Can you work these out from the model? Positions are in its coordinate system, mm. A direction names the side the tool comes from. Coordinates: 2 decimals unless noted, no trailing zeros. Order: outer loops, then holes, each group sorted by start corner. A loop starts at its lowest first (then second) coordinate and runs counter-clockwise, first axis right, second up. Notation, with made-up numbers: (6.5, -21.75) -> (52.5, -21.75) arc R10 ccw to (52.5, -7.75) -> close; hole circle Ø9 at (38, -29). An arc over 180 degrees is marked (long way). Answer in a Markdown table with one row per item. Add a question column.
1. If I drill on line 1 along X through (y, z) = (16.75, 0); line 2 along Y through (x, z) = (54, 14.5); line 3 along X through (y, z) = (32.5, 12), over which ranges is the centre line in solid material (lowest first)? Write a range as [from, to].
2. Imagine slicing it at A-A on z = 0. Write out the boundary of the cut face in (x, y), plus the area to 3 significant figures.
3. Imagine slicing it at B-B on y = 26. Write out the boundary of the cut face in (x, z).
4. Will these pins go through, and if not, where does the flat tip stop? pin 1 (11 mm diameter, centred on y = 29.5, z = -2.5, fed in from +X); pin 2 (5.5 mm diameter, centred on x = -51.96, z = 30, fed in from +Y); pin 3 (17.5 mm diameter, centred on x = 40.5, z = 33.5, fed in from +Y); pin 4 (23 mm diameter, centred on x = 0, z = 0, fed in from -Y).
5. We'd pull the mould along Z, two halves only. Please class faces 4 (the face through (-8.99, 27.93, -22.79)), 5 (the face through (25.14, 27.93, -19.684)), 6 (the face through (17, 0, -14)): pulls with the +Z half, pulls with the -Z half, needs draft (parallel to the pull), parting line crosses it, or undercut.
6. On a 3-axis mill with a long thin cutter (end or side, diameter ignored), from which of +Z, -Z, +X, -X, +Y, -Y can I reach the whole of each face in a straight line? I mean faces 1 (the face through (-1, 11, -59)), 2 (the face through (48, 33, 33)), 3 (the face through (73, 20, 8)). Say none if no direction works.
7. Imagine slicing it at D-D on z = -40. Write out the boundary of the cut face in (x, y), plus the area to 3 significant figures.
8. Imagine slicing it at C-C on x = 28. Write out the boundary of the cut face in (y, z) (3 decimals), plus the area to 3 significant figures.
from build123d import *
from build123d.topology import SkipClean

# Parameters (mm, degrees)
SKETCH_1_W                   = 160
SKETCH_1_H                   = 118
EXTRUDE_1_DEPTH              = 23
EXTRUDE_2_DEPTH              = 38
HOLE_WIZARD_M8_2_D           = 6.8
HOLE_WIZARD_M8_2_DEPTH       = 17.957073895
HOLE_WIZARD_M8_2_CSINK_D     = 8.05
HOLE_WIZARD_M8_2_CSINK_ANGLE = 90
HOLE_WIZARD_M8_2_TIP         = 2.042926105
SKETCH_6_R                   = 24.5
EXTRUDE_3_DEPTH              = 10
EXTRUDE_4_DEPTH              = 10
SKETCH_9_R                   = 19
CUT_EXTRUDE_1_DEPTH          = 105.737767782
CUT_EXTRUDE_2_DEPTH          = 6


with BuildPart() as part:
    # Sketch 1 → Extrude 1 (new body)
    with BuildSketch(Plane(origin=(0, 0, 0), x_dir=(1, 0, 0), z_dir=(0, 1, 0))):
        Rectangle(SKETCH_1_W, SKETCH_1_H)
    extrude(amount=EXTRUDE_1_DEPTH)

    # Sketch 1_3 → Extrude 2 (add)
    with BuildSketch(Plane(origin=(0, 0, 0), x_dir=(1, 0, 0), z_dir=(0, 1, 0))):
        with BuildLine():
            ThreePointArc((-64.951905284, 37.5), (-75, 0), (-64.951905284, -37.5))
            ThreePointArc((-64.951905284, -37.5), (-44.461524227, -42.990381057), (-38.97114317, -22.5))
            ThreePointArc((-38.97114317, -22.5), (-45, 0), (-38.97114317, 22.5))
            ThreePointArc((-38.97114317, 22.5), (-44.461524227, 42.990381057), (-64.951905284, 37.5))
        make_face()
    extrude(amount=EXTRUDE_2_DEPTH)

    # Hole Wizard M8 _2
    with Locations(Plane(origin=(0, 38, 0), x_dir=(1, 0, 0), z_dir=(0, 1, 0))):
        with Locations((-51.961524227, 30), (-51.961524227, -30)):
            CounterSinkHole(HOLE_WIZARD_M8_2_D / 2, HOLE_WIZARD_M8_2_CSINK_D / 2, depth=HOLE_WIZARD_M8_2_DEPTH, counter_sink_angle=HOLE_WIZARD_M8_2_CSINK_ANGLE)
            with Locations((0, 0, -(HOLE_WIZARD_M8_2_DEPTH + HOLE_WIZARD_M8_2_TIP / 2))):  # 118° drill point
                Cone(0, HOLE_WIZARD_M8_2_D / 2, HOLE_WIZARD_M8_2_TIP, mode=Mode.SUBTRACT)

    # Sketch 6 → Extrude 3 (add)
    with BuildSketch(Plane(origin=(0, 23, 0), x_dir=(1, 0, 0), z_dir=(0, 1, 0))):
        with BuildLine():
            ThreePointArc((-16.916580755, -17.722282459), (-24.5, 0), (-16.916580755, 17.722282459))
            ThreePointArc((-16.916580755, 17.722282459), (-30.649129847, 15.709991673), (-37.095262413, 28.001435595))
            ThreePointArc((-37.095262413, 28.001435595), (-37.764179884, 25.158986305), (-38.97114317, 22.5))
            ThreePointArc((-38.97114317, 22.5), (-45, 0), (-38.97114317, -22.5))
            ThreePointArc((-38.97114317, -22.5), (-37.764179884, -25.158986305), (-37.095262413, -28.001435595))
            ThreePointArc((-37.095262413, -28.001435595), (-30.649129847, -15.709991673), (-16.916580755, -17.722282459))
        make_face()
        Circle(SKETCH_6_R)
        with BuildLine():
            Line((15, 24.5), (0, 24.5))
            ThreePointArc((0, 24.5), (17.324116139, 17.324116139), (24.5, 0))
            ThreePointArc((24.5, 0), (21.217622393, -12.25), (12.25, -21.217622393))
            Line((12.25, -21.217622393), (30, -10.969655115))
            ThreePointArc((30, -10.969655115), (32.66631784, -9.127014863), (35, -6.877903594))
            Line((35, -6.877903594), (35, 0))
            Line((35, 0), (35, 15))
            Line((35, 15), (15, 24.5))
        make_face()
    extrude(amount=EXTRUDE_3_DEPTH)

    # Sketch 8 → Extrude 4 (add)
    with BuildSketch(Plane(origin=(0, 23, 0), x_dir=(1, 0, 0), z_dir=(0, 1, 0))):
        with BuildLine():
            Line((25.800739315, 36.377490991), (43.008032405, 11.802929662))
            Line((43.008032405, 11.802929662), (57.971696229, 26.766593486))
            ThreePointArc((57.971696229, 26.766593486), (59.260216754, 41.494450487), (44.979858235, 45.32086102))
            Line((44.979858235, 45.32086102), (25.800739315, 36.377490991))
        make_face()
        with BuildLine():
            Line((43.008032405, -11.802929662), (57.971696229, -26.766593486))
            ThreePointArc((57.971696229, -26.766593486), (59.260216754, -41.494450487), (44.979858235, -45.32086102))
            Line((44.979858235, -45.32086102), (25.800739315, -36.377490991))
            Line((25.800739315, -36.377490991), (43.008032405, -11.802929662))
        make_face()
    extrude(amount=EXTRUDE_4_DEPTH)

    # Sketch 9 → Cut-Extrude 1 (cut, through all)
    with BuildSketch(Plane(origin=(0, 33, 0), x_dir=(1, 0, 0), z_dir=(0, 1, 0))):
        with Locations(Location((0, 0, 0), (0, 0, 270))):
            Circle(SKETCH_9_R)
    extrude(amount=-CUT_EXTRUDE_1_DEPTH, mode=Mode.SUBTRACT)

    # Sketch 10 → Cut-Revolve 5 (revolve, cut)
    with SkipClean():  # the faces are left unmerged after this step: merging them gives an invalid solid
        with BuildSketch(Plane.XY, mode=Mode.PRIVATE) as cut_revolve_5_sk:
            with BuildLine():
                ThreePointArc((0, 83), (-30, 53), (0, 23))
                Line((0, 23), (0, 83))
            make_face()
            with BuildLine():
                Line((0, 83), (0, 23))
                ThreePointArc((0, 23), (21.213203436, 31.786796564), (30, 53))
                ThreePointArc((30, 53), (21.213203436, 74.213203436), (0, 83))
            make_face()
        revolve(cut_revolve_5_sk.sketch.rotate(Axis((0, 23, 0), (0, 1, 0)), 270), axis=Axis((0, 23, 0), (0, 1, 0)), mode=Mode.SUBTRACT)
    add(part.part.scale(1), mode=Mode.REPLACE)  # the faces are merged on a copy

    # Sketch 11 → Cut-Extrude 2 (cut)
    with BuildSketch(Plane(origin=(0, 23, 0), x_dir=(1, 0, 0), z_dir=(0, 1, 0))):
        with BuildLine():
            Line((95, -8), (65, -8))
            ThreePointArc((65, -8), (57, 0), (65, 8))
            Line((65, 8), (95, 8))
            ThreePointArc((95, 8), (103, 0), (95, -8))
        make_face()
    extrude(amount=-CUT_EXTRUDE_2_DEPTH, mode=Mode.SUBTRACT)


solid = part.part
Answers follow:
| question | item | result |
|---|---|---|
| 1 | line 1 | x = [-80, -19], [19, 80] |
| 1 | line 2 | y = [0, 23] |
| 1 | line 3 | x = [-74.03, -18.32], [18.32, 28.22], [42.87, 43.21] |
| 2 | outline | (-80, 0) -> (-19, 0) -> (-19, 29.78) arc R30 cw to (-22.36, 33) -> (-45, 33) -> (-45, 38) -> (-75, 38) -> (-75, 23) -> (-80, 23) -> close; (19, 0) -> (80, 0) -> (80, 17) -> (57, 17) -> (57, 23) -> (35, 23) -> (35, 33) -> (22.36, 33) arc R30 cw to (19, 29.78) -> close |
| 2 | area | 3,530 mm² |
| 3 | outline | (-64.95, -37.5) arc R15 ccw to (-37.1, -28) arc R12 cw to (-16.92, -17.72) arc R24.5 ccw to (0, -24.5) -> (15, -24.5) -> (35, -15) -> (35, 6.88) arc R20 ccw to (30, 10.97) -> (12.25, 21.22) arc R24.5 ccw to (-16.92, 17.72) arc R12 cw to (-37.1, 28) arc R15 ccw to (-64.95, 37.5) arc R75 ccw to start; (25.8, -36.38) -> (44.98, -45.32) arc R11.5 ccw to (57.97, -26.77) -> (43.01, -11.8) -> close; (25.8, 36.38) -> (43.01, 11.8) -> (57.97, 26.77) arc R11.5 ccw to (44.98, 45.32) -> close; hole circle Ø6.8 at (-51.96, -30); hole circle Ø6.8 at (-51.96, 30); hole circle Ø38 at (0, 0) |
| 4 | pin 1 | stops at x = 35 |
| 4 | pin 2 | stops at y = 19.65 |
| 4 | pin 3 | stops at y = 33 |
| 4 | pin 4 | passes through |
| 5 | face 4 | pulls with the -Z half |
| 5 | face 5 | undercut |
| 5 | face 6 | needs draft |
| 6 | face 1 | -Z, +X, -X, +Y, -Y |
| 6 | face 2 | +Z, -Z, +X, +Y |
| 6 | face 3 | +X, +Y |
| 7 | outline | (-80, 0) -> (80, 0) -> (80, 23) -> (60.15, 23) -> (60.15, 33) -> (33.57, 33) -> (33.57, 23) -> (-40.78, 23) -> (-40.78, 38) -> (-63.14, 38) -> (-63.14, 23) -> (-80, 23) -> close |
| 7 | area | 4,280 mm² |
| 8 | outline | (0, -59) -> (23, -59) -> (23, -37.403) -> (33, -37.403) -> (33, -33.237) -> (23, -33.237) -> (23, -18.325) -> (33, -18.325) -> (33, 12.124) -> (23, 12.124) -> (23, 33.237) -> (33, 33.237) -> (33, 37.403) -> (23, 37.403) -> (23, 59) -> (0, 59) -> close |
| 8 | area | 3,100 mm² |
